Could you check a few things on this model? Use its own coordinates, in mm. A direction names the side the tool comes from. Give positions to 0.01 mm unless a question says otherwise; leave off trailing zeros. Loops run counter-clockwise (first coordinate to the right, second up) from the corner with the lowest first, then second, coordinate; pieces in that order, holes last. Notation, with made-up numbers: M 3,68.5 L 42,68.5 A11 cw 42,78.5 Z; hole C 8,62.5 d1. An arc over 180 degrees is marked long. Return JSON: item names as keys, results as strings. Group by question number.
1. If we section it at A-A (y = 2): Write out the boundary of the cut face in (x, z).
2. For pin 1 (1.9 mm diameter, centred on x = 41.11, z = 33.1, fed in from -Y), with a flat end and sliding along its axis, tell me the tip position at first contact or that it passes through.
3. For faces 1 (the cylindrical face through (-3.965, 1.479, 37.157)), 2 (the flat face through (1, 2, 35.977)), which set-ups out of +Z, -Z, +X, -X, +Y, -Y let a thin tool reach every point of the face, with its end or its side?
4. Please list where these lines run through material, in increasing order: line 1 (X direction, y = 1.4, z = 33); line 2 (X direction, y = 0.15, z = 32.5); line 3 (Z direction, x = 41.5, y = 1.9).
5. If we mould it in two halves opening along X, with no side actions, what happens to faces 3 (the cylindrical face through (42.459, 1.521, 33.957)), 4 (the flat face through (1, 2, 31.286)), 5 (the cylindrical face through (126.675, 1.479, 37.175)), 6 (the flat face through (62, 1, 26.094))? For each: +X half, -X half, draft (parallel to the pull), parting line (faces both ways), or undercut.
```python
from build123d import *

# Parameters (mm, degrees)
BOSS_EXTRUDE1_DEPTH = 3
CUT_EXTRUDE1_DEPTH  = 1
CUT_EXTRUDE3_REACH  = 138.82
CUT_EXTRUDE4_REACH  = 138.82


with BuildPart() as part:
    # Sketch3 → Boss-Extrude1 (new body)
    with BuildSketch(Plane(origin=(0, 0, 0), x_dir=(1, 0, 0), z_dir=(0, 1, 0))):
        with BuildLine():
            Line((131.37466785, -26.093767651), (-8.62533215, -26.093767651))
            Line((-8.62533215, -26.093767651), (-8.62533215, -33.834747513))
            ThreePointArc((-8.62533215, -33.834747513), (-7.746652493, -35.956067857), (-5.62533215, -36.834747513))
            Line((-5.62533215, -36.834747513), (-5.431022837, -36.834747513))
            ThreePointArc((-5.431022837, -36.834747513), (-3.945556452, -37.165616778), (-2.74094445, -38.095667731))
            Line((-2.74094445, -38.095667731), (125.49028015, -38.095667731))
            ThreePointArc((125.49028015, -38.095667731), (126.694892152, -37.165616778), (128.180358538, -36.834747513))
            Line((128.180358538, -36.834747513), (128.37466785, -36.834747513))
            ThreePointArc((128.37466785, -36.834747513), (130.495988194, -35.956067857), (131.37466785, -33.834747513))
            Line((131.37466785, -33.834747513), (131.37466785, -26.093767651))
        make_face()
    extrude(amount=BOSS_EXTRUDE1_DEPTH)

    # Sketch4 → Cut-Extrude1 (cut)
    with BuildSketch(Plane.XZ):
        with BuildLine():
            Line((2.050442501, 32.498814854), (1.736339937, 32.498814854))
            add(Edge.make_bspline(
                [(1.736339937, 32.498814854), (1.73838709, 32.540485742), (1.742407644, 32.622326256), (1.761235933, 32.741650163), (1.78817681, 32.855704962), (1.826268264, 32.963574876), (1.873574542, 33.066213683), (1.930304569, 33.163213699), (1.99749842, 33.254204887), (2.073705154, 33.338343731), (2.156473793, 33.415531301), (2.245779732, 33.482186544), (2.33962476, 33.538504215), (2.437724159, 33.585585457), (2.541184722, 33.620925303), (2.64906758, 33.647146943), (2.761846716, 33.662923289), (2.838686738, 33.664619074), (2.877766219, 33.665481521)],
                knots=[0, 0, 0, 0, 1.10065271, 2.161652631, 3.183658789, 4.190468796, 5.17591951, 6.163126047, 7.15150782, 8.156236427, 9.156009102, 10.134482811, 11.092018607, 12.041330605, 13.001268258, 13.972401359, 14.968799086, 16, 16, 16, 16], degree=3))
            add(Edge.make_bspline(
                [(2.877766219, 33.665481521), (2.916144293, 33.664583064), (2.991555837, 33.66281763), (3.101617852, 33.6476566), (3.206395146, 33.623911009), (3.305682913, 33.590595592), (3.398688977, 33.545811165), (3.486112022, 33.492013626), (3.568992833, 33.429793795), (3.643599616, 33.356539981), (3.712107696, 33.278337597), (3.771209951, 33.194849693), (3.821823114, 33.108620408), (3.864010794, 33.018992206), (3.895066933, 32.925121178), (3.918645141, 32.828373975), (3.931972555, 32.727749164), (3.934017978, 32.659642608), (3.935057885, 32.625016777)],
                knots=[0, 0, 0, 0, 1.111607364, 2.184268762, 3.212621178, 4.221274766, 5.211760367, 6.196651075, 7.1921475, 8.207485113, 9.220403448, 10.201281604, 11.166441695, 12.114753415, 13.065576456, 14.026450734, 14.996634279, 16, 16, 16, 16], degree=3))
            add(Edge.make_bspline(
                [(3.935057885, 32.625016777), (3.93337124, 32.576266968), (3.930027549, 32.47962284), (3.901171846, 32.337418482), (3.856589749, 32.199513423), (3.80251672, 32.088534371), (3.747896152, 31.999557478), (3.699716357, 31.925641836), (3.642064004, 31.84681542), (3.575466591, 31.762284311), (3.500928784, 31.671789941), (3.417914117, 31.575295175), (3.325788426, 31.47382487), (3.261130244, 31.404519057), (3.227625994, 31.368606521)],
                knots=[0, 0, 0, 0, 1.184203166, 2.347625244, 3.513805382, 4.700623107, 5.337941753, 6.051866363, 6.845199593, 7.711357327, 8.668078039, 9.695487809, 10.805859518, 12, 12, 12, 12], degree=3))
            Line((3.227625994, 31.368606521), (2.351924872, 30.43471229))
            Line((2.351924872, 30.43471229), (3.97992968, 30.43471229))
            Line((3.97992968, 30.43471229), (3.97992968, 30.075737931))
            Line((3.97992968, 30.075737931), (1.601724552, 30.075737931))
            Line((1.601724552, 30.075737931), (2.959096347, 31.524255559))
            add(Edge.make_bspline(
                [(2.959096347, 31.524255559), (2.992144234, 31.558753866), (3.055622461, 31.625018052), (3.145405038, 31.721761013), (3.226044026, 31.811510553), (3.298061419, 31.894097102), (3.359894924, 31.97072867), (3.414767156, 32.038923373), (3.458732747, 32.101677823), (3.506448143, 32.174418437), (3.552662124, 32.263230755), (3.59237448, 32.371764444), (3.616589329, 32.483491696), (3.619494164, 32.558993734), (3.620955321, 32.596971905)],
                knots=[0, 0, 0, 0, 1.329631726, 2.553950428, 3.673215718, 4.687767853, 5.603093632, 6.413772471, 7.123043292, 7.734684054, 8.834405432, 9.900288307, 10.943827018, 12, 12, 12, 12], degree=3))
            add(Edge.make_bspline(
                [(3.620955321, 32.596971905), (3.620319579, 32.620853304), (3.619066653, 32.667918954), (3.608008955, 32.736924713), (3.591298449, 32.803489527), (3.567353191, 32.867818146), (3.535746451, 32.929263798), (3.497273071, 32.987901278), (3.452883008, 33.044590244), (3.401531739, 33.097743542), (3.345120219, 33.146424747), (3.285525969, 33.189548833), (3.222475865, 33.225587943), (3.156235743, 33.255131441), (3.086990273, 33.278306822), (3.014605528, 33.294365401), (2.939281512, 33.304447885), (2.887848016, 33.305812057), (2.861640417, 33.306507162)],
                knots=[0, 0, 0, 0, 0.991446411, 1.95395049, 2.89581595, 3.838931463, 4.798493298, 5.75982156, 6.748411868, 7.785213223, 8.824556874, 9.840280684, 10.836137867, 11.835679398, 12.848801643, 13.863922112, 14.911575587, 16, 16, 16, 16], degree=3))
            add(Edge.make_bspline(
                [(2.861640417, 33.306507162), (2.834269585, 33.30579213), (2.780517788, 33.304387924), (2.701598755, 33.29456526), (2.626312978, 33.27761942), (2.554471075, 33.254442745), (2.485951489, 33.224984197), (2.421087445, 33.188292452), (2.360024556, 33.144508959), (2.302648033, 33.094868403), (2.249784053, 33.039600801), (2.203337178, 32.977990838), (2.162753163, 32.911163423), (2.12734393, 32.839298872), (2.09858824, 32.761745092), (2.076615089, 32.678777387), (2.059228243, 32.590756006), (2.053419722, 32.529970921), (2.050442501, 32.498814854)],
                knots=[0, 0, 0, 0, 1.031018746, 2.02475058, 2.990194455, 3.934040569, 4.864654155, 5.795059489, 6.735614925, 7.690564532, 8.649604399, 9.611025574, 10.590972636, 11.591080095, 12.624614302, 13.701020113, 14.821632451, 16, 16, 16, 16], degree=3))
        make_face()
    extrude(amount=-CUT_EXTRUDE1_DEPTH, mode=Mode.SUBTRACT)

    # Sketch5 → Cut-Extrude3 (cut, up to next)
    with BuildSketch(Plane(origin=(0, 3, 0), x_dir=(1, 0, 0), z_dir=(0, 1, 0)), mode=Mode.PRIVATE) as cut_extrude3_sk1:
        with BuildLine():
            Line((-4.565790678, -35.977380503), (5.852113338, -35.977380503))
            ThreePointArc((5.852113338, -35.977380503), (6.91277351, -35.538040675), (7.352113338, -34.477380503))
            Line((7.352113338, -34.477380503), (7.352113338, -32.785571201))
            ThreePointArc((7.352113338, -32.785571201), (6.91277351, -31.724911029), (5.852113338, -31.285571201))
            Line((5.852113338, -31.285571201), (-4.565790678, -31.285571201))
            ThreePointArc((-4.565790678, -31.285571201), (-5.62645085, -31.724911029), (-6.065790678, -32.785571201))
            Line((-6.065790678, -32.785571201), (-6.065790678, -34.477380503))
            ThreePointArc((-6.065790678, -34.477380503), (-5.62645085, -35.538040675), (-4.565790678, -35.977380503))
        make_face()
    cut_extrude3_tool1 = extrude(cut_extrude3_sk1.sketch, amount=-CUT_EXTRUDE3_REACH, mode=Mode.PRIVATE) & part.part
    add(cut_extrude3_tool1.solids().sort_by_distance((0.643161, 3, 33.631476))[0], mode=Mode.SUBTRACT)

    # Sketch6 → Cut-Extrude4 (cut, up to next)
    with BuildSketch(Plane(origin=(0, 3, 0), x_dir=(1, 0, 0), z_dir=(0, 1, 0)), mode=Mode.PRIVATE) as cut_extrude4_sk1:
        with BuildLine():
            ThreePointArc((41.109797099, -31.496885933), (39.509797099, -33.096885933), (41.109797099, -34.696885933))
            ThreePointArc((41.109797099, -34.696885933), (42.709797099, -33.096885933), (41.109797099, -31.496885933))
        make_face()
    cut_extrude4_tool1 = extrude(cut_extrude4_sk1.sketch, amount=-CUT_EXTRUDE4_REACH, mode=Mode.PRIVATE) & part.part
    # Sketch6 → Cut-Extrude4 (cut, up to next)
    with BuildSketch(Plane(origin=(0, 3, 0), x_dir=(1, 0, 0), z_dir=(0, 1, 0)), mode=Mode.PRIVATE) as cut_extrude4_sk2:
        with BuildLine():
            ThreePointArc((81.109797099, -31.496885933), (79.509797099, -33.096885933), (81.109797099, -34.696885933))
            ThreePointArc((81.109797099, -34.696885933), (82.709797099, -33.096885933), (81.109797099, -31.496885933))
        make_face()
    cut_extrude4_tool2 = extrude(cut_extrude4_sk2.sketch, amount=-CUT_EXTRUDE4_REACH, mode=Mode.PRIVATE) & part.part
    add(cut_extrude4_tool1.solids().sort_by_distance((41.109797, 3, 33.096886))[0], mode=Mode.SUBTRACT)
    add(cut_extrude4_tool2.solids().sort_by_distance((81.109797, 3, 33.096886))[0], mode=Mode.SUBTRACT)


solid = part.part
```
Answer:
{
 "1": {"outline": "M -8.63,26.09 L 131.37,26.09 L 131.37,33.83 A3 ccw 128.37,36.83 L 128.18,36.83 A3.5 cw 125.49,38.1 L -2.74,38.1 A3.5 cw -5.43,36.83 L -5.63,36.83 A3 ccw -8.63,33.83 Z; hole M -6.07,32.79 A1.5 ccw -4.57,31.29 L 5.85,31.29 A1.5 ccw 7.35,32.79 L 7.35,34.48 A1.5 ccw 5.85,35.98 L -4.57,35.98 A1.5 ccw -6.07,34.48 Z; hole C 41.11,33.1 d3.2; hole C 81.11,33.1 d3.2"},
 "2": {"pin 1": "passes through"},
 "3": {"face 1": "+Z, -X, +Y, -Y", "face 2": "+Y, -Y"},
 "4": {"line 1": "x = -8.63 to -6.07, 7.35 to 39.51, 42.71 to 79.51, 82.71 to 131.37", "line 2": "x = -8.63 to -6.04, 7.32 to 39.63, 42.59 to 79.63, 82.59 to 131.37", "line 3": "z = 26.09 to 31.55, 34.65 to 38.1"},
 "5": {"face 3": "undercut", "face 4": "undercut", "face 5": "+X half", "face 6": "draft"}
}
